Check sheet for the modelled part. Datum: model origin and axes. Units: mm. A direction names the side the tool comes from. Round coordinates to 2 decimals unless told otherwise and drop trailing zeros. Write each loop counter-clockwise with the first axis right and the second up, starting at its lowest first coordinate (ties: lowest second). Pieces come first, ordered by that corner, then holes. Notation, with made-up numbers: M 24.5,3 L 47.5,3 A23 ccw 47.5,24 Z; hole C -4.5,-18.75 d8. An arc over 180 degrees is marked long. Answer in a Markdown table with one row per item.
```python
from build123d import *

# Parameters (mm, degrees)
ESQUISSE2_R             = 5
ESQUISSE2_R_2           = 1.5
ESQUISSE2_R_3           = 7.5
BOSS_EXTRU_1_DEPTH      = 16
ESQUISSE4_R             = 2
ENL_V_MAT_EXTRU_1_DEPTH = 6
ENL_V_MAT_EXTRU_2_DEPTH = 8


with BuildPart() as part:
    # Esquisse2 → Boss.-Extru.1 (new body)
    with BuildSketch(Plane.XY):
        Polygon((-56.5, 0), (56.5, 0), (56.5, 5), (44.5, 5), (44.5, 81), (-44.5, 81), (-44.5, 5), (-56.5, 5), align=None)
        with Locations(Location((-19.056527753, 21.443472247, 0), (0, 0, 180))):  # turned: the seam where the file's is
            Circle(ESQUISSE2_R, mode=Mode.SUBTRACT)
        with Locations((-19.056527753, 59.556527753)):
            Circle(ESQUISSE2_R, mode=Mode.SUBTRACT)
        with Locations(Location((19.056527753, 59.556527753, 0), (0, 0, 180))):  # turned: the seam where the file's is
            Circle(ESQUISSE2_R, mode=Mode.SUBTRACT)
        with Locations((19.056527753, 21.443472247)):
            Circle(ESQUISSE2_R, mode=Mode.SUBTRACT)
        with Locations((-41.5, 66.578130392)):
            Circle(ESQUISSE2_R_2, mode=Mode.SUBTRACT)
        with Locations(Location((41.5, 66.578130392, 0), (0, 0, 180))):  # turned: the seam where the file's is
            Circle(ESQUISSE2_R_2, mode=Mode.SUBTRACT)
        with Locations((0, 40.5)):
            Circle(ESQUISSE2_R_3, mode=Mode.SUBTRACT)
    extrude(amount=BOSS_EXTRU_1_DEPTH)

    # Esquisse4 → Enlèv. mat.-Extru.1 (cut, through all)
    with BuildSketch(Plane(origin=(0, 5, 0), x_dir=(1, 0, 0), z_dir=(0, 1, 0))):
        with Locations(Location((-51.5, -8, 0), (0, 0, 180))):  # turned: the seam where the file's is
            Circle(ESQUISSE4_R)
        with Locations((51.5, -8)):
            Circle(ESQUISSE4_R)
    extrude(amount=-ENL_V_MAT_EXTRU_1_DEPTH, mode=Mode.SUBTRACT)

    # Esquisse5 → Enlèv. mat.-Extru.2 (cut)
    with BuildSketch(Plane.XY.offset(16)):
        Polygon((-21.71636832, 69.483187891), (-28.983187891, 62.21636832), (-26.323347323, 52.289708183), (-16.396687186, 49.629867615), (-9.129867615, 56.896687186), (-11.789708183, 66.823347323), align=None)
        Polygon((-21.71636832, 11.516812109), (-28.983187891, 18.78363168), (-26.323347323, 28.710291817), (-16.396687186, 31.370132385), (-9.129867615, 24.103312814), (-11.789708183, 14.176652677), align=None)
        Polygon((26.323347323, 52.289708183), (16.396687186, 49.629867615), (9.129867615, 56.896687186), (11.789708183, 66.823347323), (21.71636832, 69.483187891), (28.983187891, 62.21636832), align=None)
        Polygon((16.396687186, 31.370132385), (9.129867615, 24.103312814), (11.789708183, 14.176652677), (21.71636832, 11.516812109), (28.983187891, 18.78363168), (26.323347323, 28.710291817), align=None)
    extrude(amount=-ENL_V_MAT_EXTRU_2_DEPTH, mode=Mode.SUBTRACT)


solid = part.part
```
1. Scan lines: L1, parallel to X at y = 41, z = 4; L2, parallel to X at y = 55, z = 5.75; L3, parallel to X at y = 16.5, z = 13. Record each from-to range of solid material in increasing order.
Found:
| item | result |
|---|---|
| L1 | x = -44.5 to -7.48, 7.48 to 44.5 |
| L2 | x = -44.5 to -21.12, -17 to 17, 21.12 to 44.5 |
| L3 | x = -44.5 to -26.7, -11.17 to 11.17, 26.7 to 44.5 |
2. Section check D-D, the plane y = 9. Record the cut outline in (x, z).
Found:
| item | result |
|---|---|
| outline | M -44.5,0 L 44.5,0 L 44.5,16 L -44.5,16 Z |
3. Go/stop test with flat-tipped pins: pin 1 (13 mm diameter, centred on x = 19.06, y = 59.56, fed in from +Z); pin 2 (5 mm diameter, centred on x = 51.5, z = 8, fed in from +Y); pin 3 (3 mm diameter, centred on y = 12, z = 5, fed in from +X). Record where each tip stops, or that it passes through.
Found:
| item | result |
|---|---|
| pin 1 | stops at z = 8 |
| pin 2 | stops at y = 5 |
| pin 3 | stops at x = 44.5 |
4. Section check C-C, the plane x = -27.5. Record the cut outline in (y, z), and give its area (3 significant figures).
Found:
| item | result |
|---|---|
| outline | M 0,0 L 81,0 L 81,16 L 63.7,16 L 63.7,8 L 56.68,8 L 56.68,16 L 24.32,16 L 24.32,8 L 17.3,8 L 17.3,16 L 0,16 Z |
| area | 1,180 mm2 |
5. Section check A-A, the plane x = 41.5. Record the cut outline in (y, z).
Found:
| item | result |
|---|---|
| outline | M 0,0 L 65.08,0 L 65.08,16 L 0,16 Z; M 68.08,0 L 81,0 L 81,16 L 68.08,16 Z |
6. Section check B-B, the plane z = 3.5. Record the cut outline in (x, y), and give its area (3 significant figures).
Found:
| item | result |
|---|---|
| outline | M -56.5,0 L 56.5,0 L 56.5,5 L 44.5,5 L 44.5,81 L -44.5,81 L -44.5,5 L -56.5,5 Z; hole C -41.5,66.58 d3; hole C -19.06,21.44 d10; hole C -19.06,59.56 d10; hole C 0,40.5 d15; hole C 19.06,21.44 d10; hole C 19.06,59.56 d10; hole C 41.5,66.58 d3 |
| area | 6,820 mm2 |
7. Access from +Z, -Z, +X, -X, +Y, -Y to the whole of each face (thin tool, end or side, straight path). Record for faces 1 (the face through (20.14, 64.438, 3.944)), 2 (the face through (-16.684, 68.135, 12.056)), 3 (the face through (44.5, 42, 8)).
Found:
| item | result |
|---|---|
| face 1 | +Z, -Z |
| face 2 | +Z |
| face 3 | +Z, -Z, +X, +Y |
8. Draft check along Z on faces 4 (the face through (24, 62, 8)), 5 (the face through (21.43, 30.02, 12.06)), 6 (the face through (50.026, 2.535, 6.648)). Enter one of: +Z half, -Z half, draft (parallel to the pull), parting line (faces both ways), or undercut.
Found:
| item | result |
|---|---|
| face 4 | +Z half |
| face 5 | draft |
| face 6 | undercut |
